Here's how the part is built. I have some questions about the finished solid (model axes, mm). A direction names the side the tool comes from. Round coordinates to 2 decimals unless told otherwise and drop trailing zeros. Write each loop counter-clockwise with the first axis right and the second up, starting at its lowest first coordinate (ties: lowest second). Pieces come first, ordered by that corner, then holes. Notation, with made-up numbers: (59, 14.5) - (97, 14.5) arc R14 ccw to (97, 35.5) - close; hole circle Ø7 at (-26, 76). An arc over 180 degrees is marked (long way). One line per item, written item: value. Start each with the question number.
Item 1: For P1, Ø5, axis at y = 42, z = 55, coming from the +X side; P2, Ø5, axis at x = 11.5, z = 125, coming from the +Y side; P3, Ø2, axis at x = -1.5, y = 33.5, coming from the -Z side, each with a flat end and sliding along its axis, tell me the tip position at first contact or that it passes through.
Item 2: If I drill on line 1 (X direction, y = 13, z = 91.5); line 2 (Y direction, x = -0.7, z = 7), over which ranges is the centre line in solid material (lowest first)?
Item 3: Thinking about a two-plate mould opening in Z: for faces 3 (the face through (-1.01, 6.94, 34.92)), 4 (the face through (-1.014, 30.536, 6.675)), 5 (the face through (-1, 20, 133)), 6 (the face through (10, 0, 66)), which applies, released by +Z, released by -Z, zero draft, split by the parting line, or undercut?
Item 4: Imagine slicing it at B-B, the plane y = 32. Please give me the cut outline in (x, z).
Item 5: Imagine slicing it at D-D, the plane y = 51. Please give me the cut outline in (x, z).
Item 6: Imagine slicing it at C-C, the plane z = 30.5. Please give me the cut outline in (x, y), then the cut area to 3 significant figures.
Item 7: Imagine slicing it at A-A, the plane z = 102.5. Please give me the cut outline in (x, y), then the cut area to 3 significant figures.
Item 8: For faces 1 (the face through (0, 31, 66)), 2 (the face through (-1.014, 40.536, 6.675)), which set-ups out of +Z, -Z, +X, -X, +Y, -Y let a thin tool reach every point of the face, with its end or its side?
```python
from build123d import *

# Parameters (mm, degrees)
SM_BASE_FLANGE_1_DEPTH = 133
CUT_EXTRUDE_1_REACH    = 149.557
SKETCH_2_R             = 6
SKETCH_2_W             = 42
SKETCH_2_H             = 22
M4X0_7_3_D             = 2.5
M4X0_7_3_DEPTH         = 7.5
M4X0_7_3_CBORE_D       = 3
M4X0_7_3_CBORE_DEPTH   = 6
M4X0_7_3_TIP           = 0.751075774
SKETCH_6_R             = 2.25
CUT_EXTRUDE_2_DEPTH    = 148.271857461


# Sheet-metal steps are written as plain solids
with BuildPart() as part:
    # Sketch 1 → 基材-凸緣1 (new body)
    with BuildSketch(Plane.XY):
        with BuildLine():
            Line((0, 60), (0, 0.7366))
            ThreePointArc((0, 0.7366), (0.215745145, 0.215745145), (0.7366, 0))
            Line((0.7366, 0), (20, 0))
            Line((20, 0), (20, -2))
            Line((20, -2), (0.7366, -2))
            ThreePointArc((0.7366, -2), (-1.198468417, -1.198468417), (-2, 0.7366))
            Line((-2, 0.7366), (-2, 60))
            Line((-2, 60), (0, 60))
        make_face()
    extrude(amount=SM_BASE_FLANGE_1_DEPTH)

    # Sketch 2 → 除料-伸長1 (cut, up to next)
    with BuildSketch(Plane.ZY.offset(2), mode=Mode.PRIVATE) as cut_extrude_1_sk1:
        with Locations((102.5, 11)):
            Circle(SKETCH_2_R)
    cut_extrude_1_tool1 = extrude(cut_extrude_1_sk1.sketch, amount=-CUT_EXTRUDE_1_REACH, mode=Mode.PRIVATE) & part.part
    # Sketch 2 → 除料-伸長1 (cut, up to next)
    with BuildSketch(Plane.ZY.offset(2), mode=Mode.PRIVATE) as cut_extrude_1_sk2:
        with Locations(Location((30.5, 11, 0), (0, 0, 180))):
            Circle(SKETCH_2_R)
    cut_extrude_1_tool2 = extrude(cut_extrude_1_sk2.sketch, amount=-CUT_EXTRUDE_1_REACH, mode=Mode.PRIVATE) & part.part
    # Sketch 2 → 除料-伸長1 (cut, up to next)
    with BuildSketch(Plane.ZY.offset(2), mode=Mode.PRIVATE) as cut_extrude_1_sk3:
        with Locations((31, 37)):
            Rectangle(SKETCH_2_W, SKETCH_2_H)
    cut_extrude_1_tool3 = extrude(cut_extrude_1_sk3.sketch, amount=-CUT_EXTRUDE_1_REACH, mode=Mode.PRIVATE) & part.part
    add(cut_extrude_1_tool1.solids().sort_by_distance((-2, 11, 102.5))[0], mode=Mode.SUBTRACT)
    add(cut_extrude_1_tool2.solids().sort_by_distance((-2, 11, 30.5))[0], mode=Mode.SUBTRACT)
    add(cut_extrude_1_tool3.solids().sort_by_distance((-2, 37, 31))[0], mode=Mode.SUBTRACT)

    # M4x0.7 螺紋孔3
    with Locations(Plane.ZY.offset(2)):
        with Locations((55, 42), (55, 32), (7, 42), (7, 32)):
            CounterBoreHole(M4X0_7_3_D / 2, M4X0_7_3_CBORE_D / 2, M4X0_7_3_CBORE_DEPTH, depth=M4X0_7_3_DEPTH)
            with Locations((0, 0, -(M4X0_7_3_DEPTH + M4X0_7_3_TIP / 2))):  # 118° drill point
                Cone(0, M4X0_7_3_D / 2, M4X0_7_3_TIP, mode=Mode.SUBTRACT)

    # 草圖6 → 除料-伸長2 (cut, through all)
    with BuildSketch(Plane(origin=(0, 0, 0), x_dir=(1, 0, 0), z_dir=(0, 1, 0))):
        with Locations(Location((11.5, -125, 0), (0, 0, 270))):
            Circle(SKETCH_6_R)
        with Locations(Location((11.5, -80, 0), (0, 0, 270))):
            Circle(SKETCH_6_R)
        with Locations(Location((11.5, -8, 0), (0, 0, 270))):
            Circle(SKETCH_6_R)
        with Locations(Location((11.5, -53, 0), (0, 0, 270))):
            Circle(SKETCH_6_R)
    extrude(amount=-CUT_EXTRUDE_2_DEPTH, mode=Mode.SUBTRACT)


solid = part.part
```
Values follow:
1. P1: stops at x = 0
1. P2: stops at y = 0
1. P3: stops at z = 0
2. line 1: x = -2 to 0
2. line 2: y = -1.59 to 30.5, 33.5 to 40.5, 43.5 to 60
3. face 3: undercut
3. face 4: undercut
3. face 5: released by +Z
3. face 6: zero draft
4. outline: (-2, 0) - (0, 0) - (0, 5.5) - (-2, 5.5) - close; (-2, 8.5) - (0, 8.5) - (0, 10) - (-2, 10) - close; (-2, 52) - (0, 52) - (0, 53.5) - (-2, 53.5) - close; (-2, 56.5) - (0, 56.5) - (0, 133) - (-2, 133) - close
5. outline: (-2, 0) - (0, 0) - (0, 133) - (-2, 133) - close
6. outline: (-2, 0.74) arc R2.74 ccw to (0.74, -2) - (20, -2) - (20, 0) - (0.74, 0) arc R0.74 cw to (0, 0.74) - (0, 5) - (-2, 5) - close; (-2, 17) - (0, 17) - (0, 26) - (-2, 26) - close; (-2, 48) - (0, 48) - (0, 60) - (-2, 60) - close
6. area: 94.5 mm^2
7. outline: (-2, 0.74) arc R2.74 ccw to (0.74, -2) - (20, -2) - (20, 0) - (0.74, 0) arc R0.74 cw to (0, 0.74) - (0, 5) - (-2, 5) - close; (-2, 17) - (0, 17) - (0, 60) - (-2, 60) - close
7. area: 139 mm^2
8. face 1: +Z, -Z, +X, +Y
8. face 2: +X, -X
